Read the model definition and answer for the solid it produces. Units are mm, in the model's axes. A direction names the side the tool comes from. Round coordinates to 2 decimals unless told otherwise and drop trailing zeros. Order: outer loops, then holes, each group sorted by start corner. A loop starts at its lowest first (then second) coordinate and runs counter-clockwise, first axis right, second up.
from build123d import *

# Parameters (mm, degrees)
BOSS_EXTRUDE1_DEPTH = 19
SKETCH4_R           = 1.980568965
CUT_EXTRUDE1_DEPTH  = 35.672179049
SKETCH6_R           = 12.5
CUT_EXTRUDE2_DEPTH  = 5


with BuildPart() as part:
    # Sketch2 → Boss-Extrude1 (new body)
    with BuildSketch(Plane(origin=(0, 0, 0), x_dir=(0, 1, 0), z_dir=(0, 0, 1))):
        with BuildLine():
            Line((10.925, 19), (-10.925, 19))
            Line((-10.925, 19), (-10.925, 14))
            Line((-10.925, 14), (-25.4, 14))
            Line((-25.4, 14), (-25.4, 0))
            Line((-25.4, 0), (-12.7, 0))
            ThreePointArc((-12.7, 0), (0, 12.7), (12.7, 0))
            Line((12.7, 0), (25.4, 0))
            Line((25.4, 0), (25.4, 14))
            Line((25.4, 14), (10.925, 14))
            Line((10.925, 14), (10.925, 19))
        make_face()
    extrude(amount=BOSS_EXTRUDE1_DEPTH)

    # Sketch4 → Cut-Extrude1 (cut, through all)
    with BuildSketch(Plane.ZY.offset(14)):
        with Locations((9.5, 19.05)):
            Circle(SKETCH4_R)
        with Locations((9.5, -19.05)):
            Circle(SKETCH4_R)
    extrude(amount=-CUT_EXTRUDE1_DEPTH, mode=Mode.SUBTRACT)

    # Sketch6 → Cut-Extrude2 (cut)
    with BuildSketch(Plane(origin=(-19, 0, 0), x_dir=(0, -1, 0), z_dir=(-1, 0, 0))):
        with Locations((-19.05, 9.5)):
            Circle(SKETCH6_R)
        with Locations((19.05, 9.5)):
            Circle(SKETCH6_R)
    extrude(amount=-CUT_EXTRUDE2_DEPTH, mode=Mode.SUBTRACT)


solid = part.part
Q1. A cutting plane is placed at A-A, the plane y = 19.05. Give the vertices of the cut face in (x, z).
Outcome:
outline: (-14, 0) - (0, 0) - (0, 7.52) - (-14, 7.52) - close; (-14, 11.48) - (0, 11.48) - (0, 19) - (-14, 19) - close
Q2. A cutting plane is placed at B-B, the plane z = 9.5. Give the vertices of the cut face in (x, y).
Outcome:
outline: (-19, -6.55) - (-14, -6.55) - (-14, -17.07) - (0, -17.07) - (0, -12.7) arc R12.7 cw to (0, 12.7) - (0, 17.07) - (-14, 17.07) - (-14, 6.55) - (-19, 6.55) - close; (-14, -25.4) - (0, -25.4) - (0, -21.03) - (-14, -21.03) - close; (-14, 21.03) - (0, 21.03) - (0, 25.4) - (-14, 25.4) - close
Q3. Straight lines are drawn through the part: probe 1 along Y at (x, z) = (-4.25, 9.5); probe 2 along Y at (x, z) = (-3.5, 10.5); probe 3 along X at (y, z) = (-21.5, 7.25). For each, find the intervals that lie inside material, in ascending order.
Outcome:
probe 1: y = -25.4 to -21.03, -17.07 to -11.97, 11.97 to 17.07, 21.03 to 25.4
probe 2: y = -25.4 to -20.76, -17.34 to -12.21, 12.21 to 17.34, 20.76 to 25.4
probe 3: x = -14 to 0
Q4. A cutting plane is placed at C-C, the plane x = -4. Give the vertices of the cut face in (y, z), plus the area to 3 significant figures.
Outcome:
outline: (-25.4, 0) - (-12.05, 0) - (-12.05, 19) - (-25.4, 19) - close; (12.05, 0) - (25.4, 0) - (25.4, 19) - (12.05, 19) - close; hole circle Ø3.96 at (-19.05, 9.5); hole circle Ø3.96 at (19.05, 9.5)
area: 483 mm2
Q5. For faces 1 (the face through (-16.54, -6.55, 9.65)), 2 (the face through (-14, 16, 9)), 3 (the face through (-7.098, 20.72, 10.565)), determine the directions among +Z, -Z, +X, -X, +Y, -Y from which every point of the face is accessible in a straight line to the end or side of a thin tool.
Outcome:
face 1: -X, -Y
face 2: -X, +Y
face 3: +X, -X
Q6. For a pull along Z with two mould halves and no side action, classify faces 4 (the face through (-12.697, -0.279, 9.367)), 5 (the face through (-14, 0, 0)), 6 (the face through (-7.1, -19.81, 11.33)), 7 (the face through (-14, 0, 19)) as released by +Z, released by -Z, zero draft, split by the parting line, or undercut.
Outcome:
face 4: zero draft
face 5: released by -Z
face 6: undercut
face 7: released by +Z
Q7. Flat-ended cylindrical pins translate along their axes: pin 1 (8 mm diameter, centred on x = -12.5, y = -11.5, fed in from -Z); pin 2 (5 mm diameter, centred on y = 15, z = 5, fed in from -X); pin 3 (2.5 mm diameter, centred on y = -19.05, z = 9.5, fed in from -X). Find the tip coordinate at first contact, or state that the pin passes through.
Outcome:
pin 1: stops at z = 0
pin 2: stops at x = -14
pin 3: passes through
Q8. A cutting plane is placed at D-D, the plane x = -13.25. Give the vertices of the cut face in (y, z).
Outcome:
outline: (-25.4, 0) - (25.4, 0) - (25.4, 19) - (-25.4, 19) - close; hole circle Ø3.96 at (-19.05, 9.5); hole circle Ø3.96 at (19.05, 9.5)
